Autodesk Inventor part; units mm, degrees
ref_plane "YZ Plane" through (0, 0, 0) normal (1, 0, 0) x (0, 1, 0)
ref_plane "XZ Plane" through (0, 0, 0) normal (0, 1, 0) x (-1, 0, 0)
ref_plane "XY Plane" through (0, 0, 0) normal (0, 0, 1) x (1, 0, 0)
sketch "スケッチ1" plane through (0, 0, 0) normal (0, 0, 1) x (1, 0, 0)
  line L0 (-7.5, -7.5) -> (7.5, -7.5)
  line L1 (7.5, -7.5) -> (7.5, 7.5)
  line L2 (7.5, 7.5) -> (-7.5, 7.5)
  line L3 (-7.5, 7.5) -> (-7.5, -7.5)
  line L4 (-7.5, -7.5) -> (7.5, 7.5) construction
  line L5 (7.5, -7.5) -> (-7.5, 7.5) construction
  point P0 (0, 0)
  dimension "d0" = 15
  dimension "d1" = 15
extrude "押し出し1" add sketch "スケッチ1" along normal blind 48
shell "シェル1" thickness 1 removed faces 2 at (-2.5, 2.5, 0) at (-2.5, 2.5, 48)
sketch "スケッチ2" plane through (-7.5, -7.5, 0) normal (0, -1, 0) x (1, 0, 0)
  line L0 (0, 0) -> (15, 0)
  point P0 (7.5, 0)
  point P1 (7.5, 7.5)
  point P2 (7.5, 0)
  point P3 (7.5, 40.5)
  point P4 (7.5, 0)
  dimension "d5" = 7.5
  dimension "d13" = 33
hole "穴1" at (0, -7.5, 7.5) at (0, -7.5, 40.5) direction (0, 1, 0) diameter 3.2 end through all
properties part number "SlideHOLDsq"
Could you check a few things on this model? Use its own coordinates, in mm. A direction names the side the tool comes from. Give positions to 0.01 mm unless a question says otherwise; leave off trailing zeros. Write each loop counter-clockwise with the first axis right and the second up, starting at its lowest first coordinate (ties: lowest second). Pieces come first, ordered by that corner, then holes. Notation, with made-up numbers: (-35, -19.75) -> (9, -19.75) arc R13 ccw to (9, 2.25) -> close; hole circle Ø11 at (61, -34.5). An arc over 180 degrees is marked (long way). Write each question's results on one line, items separated by ' | '. Start each with the question number.
Q1. I need wall thicknesses on probe 1 along Z at (x, y) = (0, -6.8); probe 2 along Y at (x, z) = (-4.5, 10.5). Which ranges of each line are inside material? Lowest first, please.
Q2. Which directions (+Z, -Z, +X, -X, +Y, -Y) give clear straight access to the entire face, cutting with the end or side of a thin tool? Please do faces 1 (the face through (0, -7.5, 24)), 2 (the face through (-6.5, 0, 24)).
Q3. Suppose I cut it at B-B, the plane y = 5.25. List the corners of the cut face in (x, z) for me, and give its area (3 significant figures).
Q4. Suppose I cut it at A-A, the plane z = 40.5. List the corners of the cut face in (x, y) for me.
Q5. I'm going to push flat-ended pins straight in: pin 1 Ø1.5 at (x, y) = (-5.5, 1.5) entering from -Z; pin 2 Ø5 at (x, z) = (0, 40.5) entering from +Y. Where does each tip first touch, or does it pass through?
Q6. We'd pull the mould along Z, two halves only. Please class faces 3 (the face through (-7, 0, 48)), 4 (the face through (0, 6.5, 24)), 5 (the face through (-1.08, 7.01, 41.68)): +Z half, -Z half, draft (parallel to the pull), parting line (faces both ways), or undercut.
Q7. Suppose I cut it at C-C, the plane x = 0. List the corners of the cut face in (y, z) for me, and give its area (3 significant figures).
Outcome:
1) probe 1: 0 to 5.9, 9.1 to 38.9, 42.1 to 48 | probe 2: -7.5 to -6.5, 6.5 to 7.5
2) face 1: +Z, -Z, +X, -X, -Y | face 2: +Z, -Z
3) outline: (-7.5, 0) -> (-6.5, 0) -> (-6.5, 48) -> (-7.5, 48) -> close; (6.5, 0) -> (7.5, 0) -> (7.5, 48) -> (6.5, 48) -> close | area: 96.0 mm2
4) outline: (-7.5, -7.5) -> (-1.6, -7.5) -> (-1.6, -6.5) -> (-6.5, -6.5) -> (-6.5, 6.5) -> (-1.6, 6.5) -> (-1.6, 7.5) -> (-7.5, 7.5) -> close; (1.6, -7.5) -> (7.5, -7.5) -> (7.5, 7.5) -> (1.6, 7.5) -> (1.6, 6.5) -> (6.5, 6.5) -> (6.5, -6.5) -> (1.6, -6.5) -> close
5) pin 1: through | pin 2: y = 7.5
6) face 3: +Z half | face 4: draft | face 5: undercut
7) outline: (-7.5, 0) -> (-6.5, 0) -> (-6.5, 5.9) -> (-7.5, 5.9) -> close; (-7.5, 9.1) -> (-6.5, 9.1) -> (-6.5, 38.9) -> (-7.5, 38.9) -> close; (-7.5, 42.1) -> (-6.5, 42.1) -> (-6.5, 48) -> (-7.5, 48) -> close; (6.5, 0) -> (7.5, 0) -> (7.5, 5.9) -> (6.5, 5.9) -> close; (6.5, 9.1) -> (7.5, 9.1) -> (7.5, 38.9) -> (6.5, 38.9) -> close; (6.5, 42.1) -> (7.5, 42.1) -> (7.5, 48) -> (6.5, 48) -> close | area: 83.2 mm2
